Check sheet for the modelled part. Datum: model origin and axes. Units: mm. Give positions to 0.01 mm unless a question says otherwise; leave off trailing zeros. Loops run counter-clockwise (first coordinate to the right, second up) from the corner with the lowest first, then second, coordinate; pieces in that order, holes last. Notation, with made-up numbers: M 54.5,25 L 101.5,25 A30 ccw 101.5,52 Z; hole C 44.5,29 d9. An arc over 180 degrees is marked long. Use one line per item in the form item = value.
Autodesk Inventor part; units mm, degrees
ref_plane "YZ Plane" through (0, 0, 0) normal (1, 0, 0) x (0, 1, 0)
ref_plane "XZ Plane" through (0, 0, 0) normal (0, 1, 0) x (-1, 0, 0)
ref_plane "XY Plane" through (0, 0, 0) normal (0, 0, 1) x (1, 0, 0)
sketch "Sketch1" plane through (0, 0, 0) normal (0, 0, 1) x (1, 0, 0)
  circle A0 centre (0, 0) radius 15.2
  circle A1 centre (0, 0) radius 3.5
  line L0 (-2.5, -2.4495) -> (2.5, -2.4495)
  dimension "d0" = 30.4
  dimension "d1" = 7
  dimension "d2" = 5
extrude "Extrusion1" add sketch "Sketch1" along normal blind 12 contours A0 | L0 A1 picked at (0.6279, -2.6163)
fillet "Fillet1" radius 2 2 edges at (-15.2, 0, 12) (-15.2, 0, 0)
1) Section check C-C (z = 10.5). Record the cut outline in (x, y).
Evaluation:
outline = C 0,0 d30.27; hole M -2.5,-2.45 L 2.5,-2.45 A3.5 ccw long Z
2) Section check A-A (y = 0). Record the cut outline in (x, z), then the cut area to 3 significant figures.
Evaluation:
outline = M -15.2,2 A2 ccw -13.2,0 L -3.5,0 L -3.5,12 L -13.2,12 A2 ccw -15.2,10 Z; M 3.5,0 L 13.2,0 A2 ccw 15.2,2 L 15.2,10 A2 ccw 13.2,12 L 3.5,12 Z
area = 277 mm^2
3) Scan lines: line 1 (Y direction, x = 0, z = 9); line 2 (Y direction, x = -1, z = 2.25); line 3 (X direction, y = -2, z = 9.75). Record each from-to range of solid material in increasing order.
Evaluation:
line_1 = -15.2 to -2.45, 3.5 to 15.2
line_2 = -15.17 to -2.45, 3.35 to 15.17
line_3 = -15.07 to -2.87, 2.87 to 15.07
4) Depth check by flat-ended pin: pin 1 Ø2.5 at (x, z) = (0.5, 8) entering from +Y; pin 2 Ø1 at (x, z) = (-2.5, 8.5) entering from -Y; pin 3 Ø1 at (y, z) = (5, 5.5) entering from -X; pin 4 Ø3 at (y, z) = (9.5, 9) entering from -X. Enter the tip coordinate at first touch or a pass-through.
Evaluation:
pin_1 = 15.2
pin_2 = -15.07
pin_3 = -14.52
pin_4 = -12.92
5) Section check B-B (z = 6.5). Record the cut outline in (x, y), then the cut area to 3 significant figures.
Evaluation:
outline = C 0,0 d30.4; hole M -2.5,-2.45 L 2.5,-2.45 A3.5 ccw long Z
area = 691 mm^2
6) Release check for a two-part mould opening along Y. For faces 1 (the face through (0, -3, 12)), 2 (the face through (0, -2.45, 6)), 3 (the face through (-0.1, 3.5, 5.9)), 4 (the face through (-15.185, -0.668, 5.944)) record: pulls with the +Y half, pulls with the -Y half, needs draft (parallel to the pull), parting line crosses it, or undercut.
Evaluation:
face_1 = needs draft
face_2 = undercut
face_3 = undercut
face_4 = parting line crosses it
